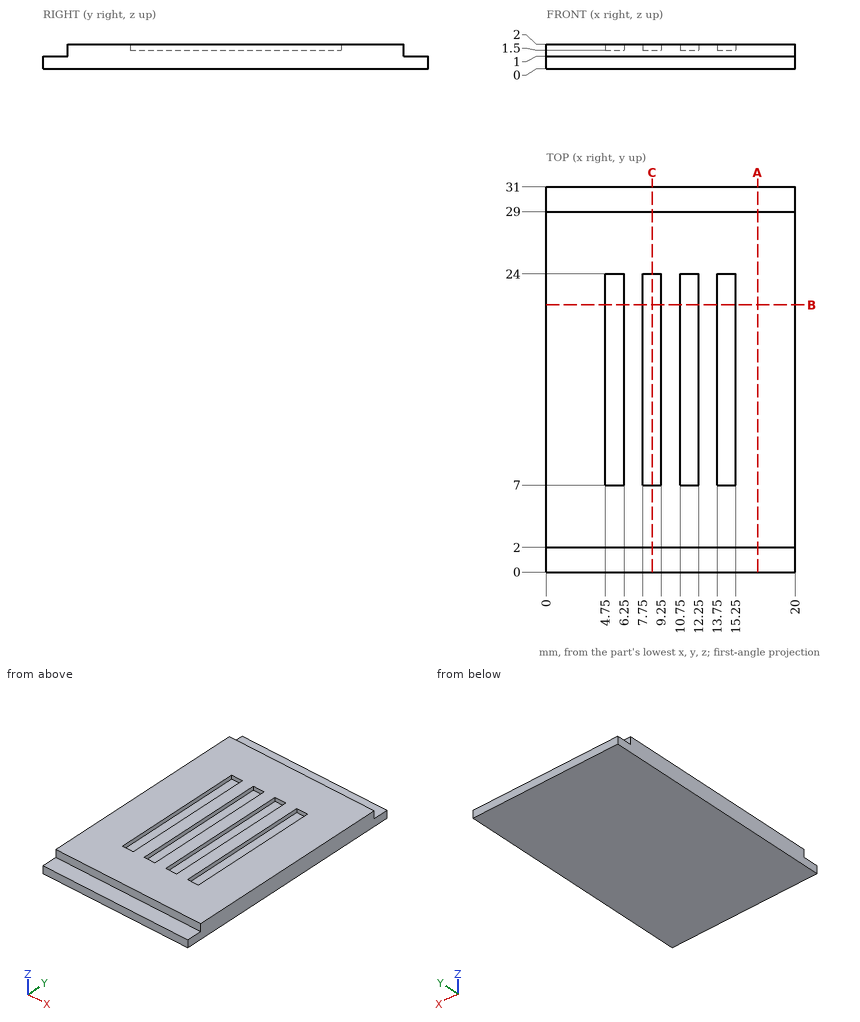
Input: dimensioned drawing with shaded views. Units: mm. Origin: part minimum x, y, z. Coordinates: 2 decimals unless noted, no trailing zeros. Order: outer loops, then holes, each group sorted by start corner. A loop starts at its lowest first (then second) coordinate and runs counter-clockwise, first axis right, second up. Notation, with made-up numbers: M 74.5,74.5 L 84.5,74.5 A20 cw 84.5,90.5 Z; hole C -32.5,-33 d8. An arc over 180 degrees is marked long. Write each question's results on one line, items separated by ' | '. Start each with the question number.
Item 1: First-contact query: pin 1 Ø1.6 at (x, y) = (6, 30.5) entering from +Z; pin 2 Ø0.6 at (x, z) = (11.5, 2) entering from -Y. Flat tips, straight axial feed; report the tip coordinate or a pass-through.
Item 2: Line query: probe 1 along X at (y, z) = (16.5, 1.85); probe 2 along Y at (x, z) = (15, 1.6); probe 3 along Y at (x, z) = (4, 1.8). Output: solid intervals per line, ascending.
Item 3: Cut plane C-C (x = 8.5). Return loops of the section in (y, z), and give its area (3 significant figures).
Item 4: Cut plane A-A (x = 17). Return loops of the section in (y, z).
Item 5: Cut plane B-B (y = 21.5). Return loops of the section in (x, z).
Checked values:
1) pin 1: stops at z = 1 | pin 2: stops at y = 2
2) probe 1: x = 0 to 4.75, 6.25 to 7.75, 9.25 to 10.75, 12.25 to 13.75, 15.25 to 20 | probe 2: y = 2 to 7, 24 to 29 | probe 3: y = 2 to 29
3) outline: M 0,0 L 31,0 L 31,1 L 29,1 L 29,2 L 24,2 L 24,1.5 L 7,1.5 L 7,2 L 2,2 L 2,1 L 0,1 Z | area: 49.5 mm2
4) outline: M 0,0 L 31,0 L 31,1 L 29,1 L 29,2 L 2,2 L 2,1 L 0,1 Z
5) outline: M 0,0 L 20,0 L 20,2 L 15.25,2 L 15.25,1.5 L 13.75,1.5 L 13.75,2 L 12.25,2 L 12.25,1.5 L 10.75,1.5 L 10.75,2 L 9.25,2 L 9.25,1.5 L 7.75,1.5 L 7.75,2 L 6.25,2 L 6.25,1.5 L 4.75,1.5 L 4.75,2 L 0,2 Z
